Build history of the part. All positions in model axes, mm. Give positions to 0.01 mm unless a question says otherwise; leave off trailing zeros. Put each result on its own line as item: value. Start each with the question number.
Item 1: Slice it at A-A, the plane z = -2.5. Give the number of separate pieces and of enclosed holes in the cut face, plus the area to 3 significant figures.
Item 2: Flat gauge pin, fed straight in: pin 1 Ø2.5 at (x, y) = (-139.7, 13.589) entering from -Z. Where does the tip first touch, or does it go through?
Item 3: Drill centre lines: line 1 along X through (y, z) = (14, -3.75) (3 decimals); line 2 along X through (y, z) = (1.5, -2.25) (3 decimals); line 3 along Y through (x, z) = (-139.7, -4) (3 decimals). Where is each one in solid material? Low to high.
Autodesk Inventor part; units mm, degrees
ref_plane "YZ Plane" through (0, 0, 0) normal (1, 0, 0) x (0, 1, 0)
ref_plane "XZ Plane" through (0, 0, 0) normal (0, 1, 0) x (-1, 0, 0)
sketch "Sketch1" plane through (0, 0, 0) normal (0, 0, 1) x (1, 0, 0)
  line L0 (0, 35.433) -> (0, -17.018)
  line L1 (-250.825, 0) -> (260.35, 0)
  line L2 (187.325, -9.525) -> (-177.8, -9.525)
  line L3 (-177.8, -9.525) -> (-177.8, 27.94)
  line L4 (-177.8, 27.94) -> (187.325, 27.94)
  line L5 (187.325, 27.94) -> (187.325, -9.525)
  point P0 (0, 0)
  point P1 (-171.45, 0)
  point P2 (0, 0)
  point P3 (63.5, 0)
  point P4 (171.45, 0)
  point P5 (-139.7, 13.589)
  point P6 (-117.475, 13.589)
  dimension "d0" = 171.45
  dimension "d1" = 63.5
  dimension "d17" = 27.94
  dimension "d18" = 9.525
  dimension "d19" = 6.35
  dimension "d20" = 187.325
  dimension "d21" = 171.45
  dimension "d33" = 22.225
  dimension "d34" = 14.351
  dimension "d35" = 38.1
extrude "Extrusion1" add sketch "Sketch1" against normal blind 6.35
sketch "Sketch2" plane through (0, 0, -6.35) normal (0, 0, -1) x (-1, 0, 0)
  point P0 (0, 0)
  point P1 (171.45, 0)
  point P2 (0, 0)
  point P3 (-63.5, 0)
  point P4 (-171.45, 0)
chamfer "Chamfer1" distance 25.4 angle 20 1 edges at (-177.8, 27.94, -3.175) measured on face at (-56.0917, 27.94, -2.1167)
fillet "Fillet1" radius 3.175 5 edges at (187.325, 27.94, -3.175) (187.325, -9.525, -3.175) (-177.8, -9.525, -3.175) (-177.8, 18.6952, -3.175) (-152.4, 27.94, -3.175)
hole "Hole2" [suppressed]
sketch "Sketch3" plane through (0, 0, 0) normal (0, 0, 1) x (1, 0, 0)
  line L0 (-171.45, -1.5875) -> (-171.45, 1.5875) construction
  line L1 (-168.91, -1.5875) -> (-168.91, 1.5875)
  line L2 (-173.99, 1.5875) -> (-173.99, -1.5875)
  arc A0 (-173.99, -1.5875) -> (-168.91, -1.5875) centre (-171.45, -1.5875) ccw
  arc A1 (-168.91, 1.5875) -> (-173.99, 1.5875) centre (-171.45, 1.5875) ccw
  line L3 (0, -1.5875) -> (0, 1.5875) construction
  line L4 (2.54, -1.5875) -> (2.54, 1.5875)
  line L5 (-2.54, 1.5875) -> (-2.54, -1.5875)
  arc A2 (-2.54, -1.5875) -> (2.54, -1.5875) centre (0, -1.5875) ccw
  arc A3 (2.54, 1.5875) -> (-2.54, 1.5875) centre (0, 1.5875) ccw
  line L6 (63.5, -1.5875) -> (63.5, 1.5875) construction
  line L7 (66.04, -1.5875) -> (66.04, 1.5875)
  line L8 (60.96, 1.5875) -> (60.96, -1.5875)
  arc A4 (60.96, -1.5875) -> (66.04, -1.5875) centre (63.5, -1.5875) ccw
  arc A5 (66.04, 1.5875) -> (60.96, 1.5875) centre (63.5, 1.5875) ccw
  line L9 (171.45, -1.5875) -> (171.45, 1.5875) construction
  line L10 (173.99, -1.5875) -> (173.99, 1.5875)
  line L11 (168.91, 1.5875) -> (168.91, -1.5875)
  arc A6 (168.91, -1.5875) -> (173.99, -1.5875) centre (171.45, -1.5875) ccw
  arc A7 (173.99, 1.5875) -> (168.91, 1.5875) centre (171.45, 1.5875) ccw
  point P0 (0, 0)
  point P1 (-171.45, 0)
  point P2 (0, 0)
  point P3 (63.5, 0)
  point P4 (171.45, 0)
  dimension "d29" = 2.54
  dimension "d30" = 3.175
extrude "Extrusion2" cut sketch "Sketch3" against normal up to next
hole "Hole3" at (-139.7, 13.589, 0) at (-117.475, 13.589, 0) direction (0, 0, -1) diameter 3.1242 end through all
Values follow:
1. separate pieces: 1
1. enclosed holes: 6
1. area: 13,400 mm2
2. pin 1: through
3. line 1: -177.8 to -141.207, -138.193 to -118.982, -115.968 to 187.325
3. line 2: -177.8 to -173.99, -168.91 to -2.54, 2.54 to 60.96, 66.04 to 168.91, 173.99 to 187.325
3. line 3: -9.525 to 12.027, 15.151 to 27.94
